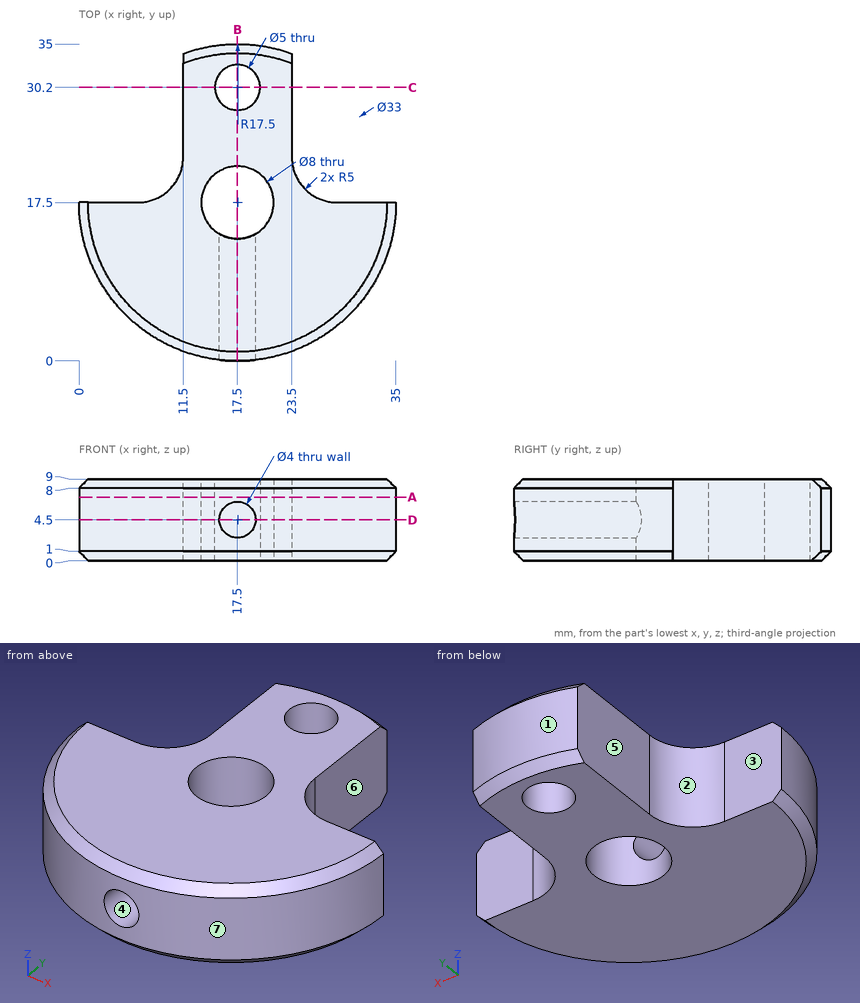
Part print with two shaded views. Sizes in mm from the minimum x, y, z corner. A direction names the side the tool comes from. Coordinates: 2 decimals unless noted, no trailing zeros. Write each loop counter-clockwise with the first axis right and the second up, starting at its lowest first coordinate (ties: lowest second). Pieces come first, ordered by that corner, then holes. Notation, with made-up numbers: M 72,41 L 128,41 A32 ccw 128,75 Z; hole C -39,-20.75 d11. An arc over 180 degrees is marked long. Return JSON: item names as keys, results as strings.
Item 1: Slice it at B-B, the plane x = 17.5. Write the cut outline in (y, z), and give its area (3 significant figures).
Findings below:
{"outline": "M 0,1 L 1,0 L 13.5,0 L 13.5,2.5 L 0,2.5 Z; M 0,6.5 L 13.5,6.5 L 13.5,9 L 1,9 L 0,8 Z; M 21.5,0 L 27.7,0 L 27.7,9 L 21.5,9 Z; M 32.7,0 L 34,0 L 35,1 L 35,8 L 34,9 L 32.7,9 Z", "area": "142 mm2"}
Item 2: Which spindle directions (+Z, -Z, +X, -X, +Y, -Y) get a long thin tool onto all of the face, cutting with end or side? Do the marked faces 5, 6 and 7. Say none if no direction does.
Findings below:
{"face 5": "+Z, -Z, -X, +Y", "face 6": "+Z, -Z, +X, +Y", "face 7": "+Z, -Z, -Y"}
Item 3: Slice it at C-C, the plane y = 30.2. Write the cut outline in (x, z), and give its area (3 significant figures).
Findings below:
{"outline": "M 11.5,0 L 15,0 L 15,9 L 11.5,9 Z; M 20,0 L 23.5,0 L 23.5,9 L 20,9 Z", "area": "63.0 mm2"}
Item 4: Probe line 1 (Y direction, x = 14, z = 5.75); line 2 (X direction, y = 5.5, z = 3.75); line 3 (X direction, y = 13.5, z = 2.75). List the from-to ranges inside material, lowest first. Write a range as from..to.
Findings below:
{"line 1": "y = 0.35..15.56, 19.44..34.65", "line 2": "x = 4.76..15.65, 19.35..30.24", "line 3": "x = 0.46..16.53, 18.47..34.54"}
Item 5: Two-plate mould, pull along X, no slides. Class the marked faces 1, 2, 3 and 4: +X half, -X half, draft (parallel to the pull), parting line (faces both ways), or undercut.
Findings below:
{"face 1": "parting line", "face 2": "-X half", "face 3": "draft", "face 4": "undercut"}
Item 6: Slice it at A-A, the plane z = 7. Write the cut outline in (x, y).
Findings below:
{"outline": "M 0,17.5 A17.5 ccw 35,17.5 L 28.5,17.5 A5 cw 23.5,22.5 L 23.5,33.94 A17.5 ccw 11.5,33.94 L 11.5,22.5 A5 cw 6.5,17.5 Z; hole C 17.5,17.5 d8; hole C 17.5,30.2 d5"}
Item 7: Slice it at D-D, the plane z = 4.5. Write the cut outline in (x, y), and give its area (3 significant figures).
Findings below:
{"outline": "M 0,17.5 A17.5 ccw 15.5,0.11 L 15.5,14.04 A4 cw long 19.5,14.04 L 19.5,0.11 A17.5 ccw 35,17.5 L 28.5,17.5 A5 cw 23.5,22.5 L 23.5,33.94 A17.5 ccw 11.5,33.94 L 11.5,22.5 A5 cw 6.5,17.5 Z; hole C 17.5,30.2 d5", "area": "573 mm2"}
Item 8: Drop flat-ended pins along their axis: pin 1 Ø4 at (x, z) = (22.5, 3) entering from -Y; pin 2 Ø2.5 at (y, z) = (27.5, 4) entering from -X; pin 3 Ø2 at (x, z) = (8.5, 3) entering from -Y. Give the stop position or say it passes through.
Findings below:
{"pin 1": "stops at y = 0.26", "pin 2": "stops at x = 11.5", "pin 3": "stops at y = 1.94"}
